from build123d import *

# Parameters (mm, degrees)
SKETCH1_R      = 5.9
EXTRUDE1_DEPTH = 51
SKETCH2_R      = 4.263277526
EXTRUDE2_DEPTH = 52.678041759
FILLET1_R      = 0.4
SKETCH3_W      = 0.324130055
SKETCH3_H      = 0.237695373


with BuildPart() as part:
    # Sketch1 → Extrude1 (new body)
    with BuildSketch(Plane.XY):
        Circle(SKETCH1_R)
    extrude(amount=EXTRUDE1_DEPTH)

    # Sketch2 → Extrude2 (cut, through all)
    with BuildSketch(Plane.XY.offset(51)):
        Circle(SKETCH2_R)
    extrude(amount=-EXTRUDE2_DEPTH, mode=Mode.SUBTRACT)

    # Fillet1
    fillet1_edges = [part.edges().sort_by_distance(p)[0] for p in [
        (-5.9, 0, 0),
        (-5.9, 0, 51),
        (-4.263277526, 0, 0),
        (-4.263277526, 0, 51),
    ]]
    fillet(fillet1_edges, radius=FILLET1_R)

    # Cut-Sweep2: sweep along a curve in space
    with BuildLine() as cut_sweep2_path:
        ThreePointArc((4.263277526, 0, 0.4), (3.014592449, 3.014592449, 0.4), (0, 4.263277526, 0.4))
        ThreePointArc((0, 4.263277526, 0.4), (-3.014592449, 3.014592449, 0.4), (-4.263277526, 0, 0.4))
        ThreePointArc((-4.263277526, 0, 0.4), (-3.014592449, -3.014592449, 0.4), (0, -4.263277526, 0.4))
        ThreePointArc((0, -4.263277526, 0.4), (3.014592449, -3.014592449, 0.4), (4.263277526, 0, 0.4))
    # Sketch3 → Cut-Sweep2 (sweep, cut)
    with BuildSketch(Plane(origin=(0, 0, 0), x_dir=(1, 0, 0), z_dir=(0, 1, 0))):
        with Locations((-4.241785701, -0.709092592)):
            Rectangle(SKETCH3_W, SKETCH3_H)
    sweep(path=cut_sweep2_path.line, mode=Mode.SUBTRACT)


solid = part.part
Check sheet for the modelled part. Datum: model origin and axes. Units: mm. Give positions to 0.01 mm unless a question says otherwise; leave off trailing zeros. Write each loop counter-clockwise with the first axis right and the second up, starting at its lowest first coordinate (ties: lowest second). Pieces come first, ordered by that corner, then holes. Notation, with made-up numbers: (-27, 89.25) -> (-5, 89.25) arc R13 ccw to (-5, 104.25) -> close; hole circle Ø10 at (4.5, 42). An arc over 180 degrees is marked (long way). One line per item, written item: value. Start each with the question number.
Item 1: Material ranges on probe 1 along Y at (x, z) = (0, 0.55); probe 2 along X at (y, z) = (1.25, 36.5); probe 3 along X at (y, z) = (-0.25, 49.5), recorded low to high. Write a range as from..to.
Item 2: Draft check along X on faces 1 (the cylindrical face through (-5.894, 0.259, 25.149)), 2 (the cylindrical face through (-3.142, 2.881, 26.062)), 3 (the flat face through (-4, 3, 0)). Enter one of: +X half, -X half, draft (parallel to the pull), parting line (faces both ways), or undercut.
Item 3: Gauge pin test, flat ends, axial feed: pin 1 (1 mm diameter, centred on x = 2, z = 5, fed in from -Y); pin 2 (2 mm diameter, centred on y = 4.5, z = 37, fed in from +X); pin 3 (2 mm diameter, centred on x = -2.5, z = 27.5, fed in from +Y). Record the tip position at first contact, or that the pin passes through.
Item 4: Section check A-A on z = 47. Record the cut outline in (x, y), then the cut area to 3 significant figures.
Results list:
1. probe 1: -5.9..-4.26, 4.26..5.9
1. probe 2: -5.77..-4.08, 4.08..5.77
1. probe 3: -5.89..-4.26, 4.26..5.89
2. face 1: parting line
2. face 2: undercut
2. face 3: draft
3. pin 1: y = -5.71
3. pin 2: x = 4.75
3. pin 3: y = 5.71
4. outline: circle Ø11.8 at (0, 0); hole circle Ø8.53 at (0, 0)
4. area: 52.3 mm²
